```python
from build123d import *

# Parameters (mm, degrees)
SKETCH1_R           = 19.05
SKETCH1_R_2         = 4
BOSS_EXTRUDE1_DEPTH = 47.498
SKETCH1_3_R         = 4
BOSS_EXTRUDE2_DEPTH = 55.498


with BuildPart() as part:
    # Sketch1 → Boss-Extrude1 (new, symmetric)
    # profile 1 of 2: a face of its own
    with BuildSketch(Plane.XY):
        with Locations(Location((0, 0, 0), (0, 0, 180))):
            Circle(SKETCH1_R)
        Circle(SKETCH1_R_2, mode=Mode.SUBTRACT)
    # profile 2 of 2: a face of its own
    with BuildSketch(Plane.XY):
        Circle(SKETCH1_R_2)
    extrude(amount=BOSS_EXTRUDE1_DEPTH, both=True)

    # Sketch1_3 → Boss-Extrude2 (add, symmetric)
    with BuildSketch(Plane.XY):
        Circle(SKETCH1_3_R)
    extrude(amount=BOSS_EXTRUDE2_DEPTH, both=True)


solid = part.part
```
CAD build for the part. Positions are in the model's coordinates, mm. A direction names the side the tool comes from. Coordinates: 2 decimals unless noted, no trailing zeros. Write each loop counter-clockwise with the first axis right and the second up, starting at its lowest first coordinate (ties: lowest second). Pieces come first, ordered by that corner, then holes. Notation, with made-up numbers: (-19.75, -26) -> (31.25, -26) arc R20 cw to (31.25, -16) -> close; hole circle Ø3 at (5.5, -8). An arc over 180 degrees is marked (long way). Use CSV: the item, a comma, the result in double quotes. Start each with the question number.
Item 1: Wall check: probe 1 along Z at (x, y) = (9.5, 2.5); probe 2 along X at (y, z) = (-0.5, -16); probe 3 along X at (y, z) = (-10, -36). Give the ranges that are in metal, low to high.
Item 2: Band-saw the part on C-C, the plane z = -7. Write the cut outline in (x, y).
Item 3: Tool access for faces 1 (the cylindrical face through (-0.867, -3.905, 51.554)), 2 (the cylindrical face through (-0.867, -3.905, -51.442)), 3 (the flat face through (0, 0, 55.498)): list every direction of +Z, -Z, +X, -X, +Y, -Y with a clear straight run to the whole face (end or side of a thin tool).
Item 4: Band-saw the part on A-A, the plane x = 0. Write the cut outline in (y, z).
Item 5: Drop flat-ended pins along their axis: P1, Ø2, axis at y = 7.5, z = -1.5, coming from the -X side; P2, Ø2, axis at y = 6, z = -33, coming from the -X side; P3, Ø6, axis at x = 10, z = -21.5, coming from the +Y side. Give the stop position or say it passes through.
Item 6: Band-saw the part on D-D, the plane x = 17. Write the cut outline in (y, z).
Response values:
1,probe 1,"z = -47.5 to 47.5"
1,probe 2,"x = -19.04 to 19.04"
1,probe 3,"x = -16.21 to 16.21"
2,outline,"circle Ø38.1 at (0, 0)"
3,face 1,"+Z"
3,face 2,"-Z"
3,face 3,"+Z, +X, -X, +Y, -Y"
4,outline,"(-19.05, -47.5) -> (-4, -47.5) -> (-4, -55.5) -> (4, -55.5) -> (4, -47.5) -> (19.05, -47.5) -> (19.05, 47.5) -> (4, 47.5) -> (4, 55.5) -> (-4, 55.5) -> (-4, 47.5) -> (-19.05, 47.5) -> close"
5,P1,"stops at x = -17.91"
5,P2,"stops at x = -18.38"
5,P3,"stops at y = 17.72"
6,outline,"(-8.6, -47.5) -> (8.6, -47.5) -> (8.6, 47.5) -> (-8.6, 47.5) -> close"
